Build history of the part. All positions in model axes, mm. Round coordinates to 2 decimals unless told otherwise and drop trailing zeros. Loops run counter-clockwise (first coordinate to the right, second up) from the corner with the lowest first, then second, coordinate; pieces in that order, holes last.
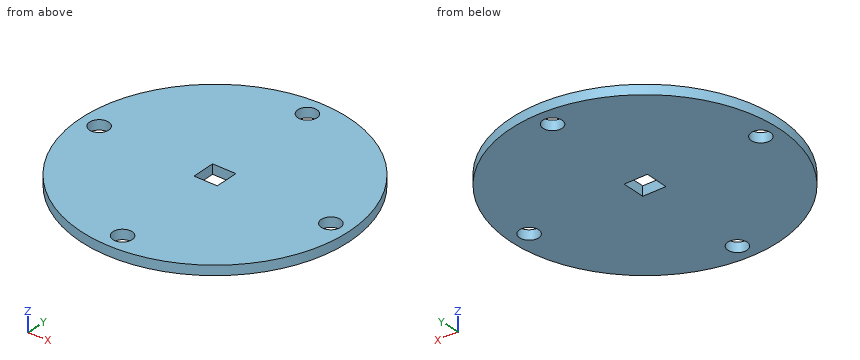
from build123d import *

# Parameters (mm, degrees)
SKETCH1_R           = 70
SKETCH1_R_2         = 5
SKETCH1_W           = 12.1
SKETCH1_H           = 12.1
BOSS_EXTRUDE1_DEPTH = 5


with BuildPart() as part:
    # Sketch1 → Boss-Extrude1 (new body)
    with BuildSketch(Plane.XY):
        Circle(SKETCH1_R)
        with Locations((0, 60.31)):
            Circle(SKETCH1_R_2, mode=Mode.SUBTRACT)
        with Locations((60.31, 0)):
            Circle(SKETCH1_R_2, mode=Mode.SUBTRACT)
        with Locations((0, -60.31)):
            Circle(SKETCH1_R_2, mode=Mode.SUBTRACT)
        with Locations((-60.31, 0)):
            Circle(SKETCH1_R_2, mode=Mode.SUBTRACT)
        with Locations((0.05, -0.1)):
            Rectangle(SKETCH1_W, SKETCH1_H, mode=Mode.SUBTRACT)
    extrude(amount=BOSS_EXTRUDE1_DEPTH)


solid = part.part
(1) Slice it at B-B on x = 0. List the corners of the cut face in (y, z).
Responses:
outline: (-70, 0) - (-65.31, 0) - (-65.31, 5) - (-70, 5) - close; (-55.31, 0) - (-6.15, 0) - (-6.15, 5) - (-55.31, 5) - close; (5.95, 0) - (55.31, 0) - (55.31, 5) - (5.95, 5) - close; (65.31, 0) - (70, 0) - (70, 5) - (65.31, 5) - close
(2) Pin check, flat tips, straight feed: P1, Ø2, axis at x = 18, z = 2.5, coming from the -Y side; P2, Ø3, axis at x = 56, z = 1, coming from the +Y side; P3, Ø1.5, axis at x = 1, z = 2.5, coming from the +Y side. Stop position of each tip, or through.
Responses:
P1: stops at y = -67.9
P2: stops at y = 43.93
P3: stops at y = 70
(3) Slice it at D-D on y = -60.31. List the corners of the cut face in (x, z).
Responses:
outline: (-35.53, 0) - (-5, 0) - (-5, 5) - (-35.53, 5) - close; (5, 0) - (35.53, 0) - (35.53, 5) - (5, 5) - close
(4) Slice it at A-A on y = 0. List the corners of the cut face in (x, z).
Responses:
outline: (-70, 0) - (-65.31, 0) - (-65.31, 5) - (-70, 5) - close; (-55.31, 0) - (-6, 0) - (-6, 5) - (-55.31, 5) - close; (6.1, 0) - (55.31, 0) - (55.31, 5) - (6.1, 5) - close; (65.31, 0) - (70, 0) - (70, 5) - (65.31, 5) - close
(5) Probe line 1 (Y direction, x = 0, z = 2.95); line 2 (Y direction, x = 60.31, z = 3.95); line 3 (X direction, y = -58, z = 0.75). List the from-to ranges inside material, lowest first.
Responses:
line 1: y = -70 to -65.31, -55.31 to -6.15, 5.95 to 55.31, 65.31 to 70
line 2: y = -35.53 to -5, 5 to 35.53
line 3: x = -39.19 to -4.43, 4.43 to 39.19
(6) Slice it at C-C on z = 2.7. List the corners of the cut face in (x, y), plus the area to 3 significant figures.
Responses:
outline: circle Ø140 at (0, 0); hole circle Ø10 at (-60.31, 0); hole (-6, -6.15) - (6.1, -6.15) - (6.1, 5.95) - (-6, 5.95) - close; hole circle Ø10 at (0, -60.31); hole circle Ø10 at (0, 60.31); hole circle Ø10 at (60.31, 0)
area: 14,900 mm2
